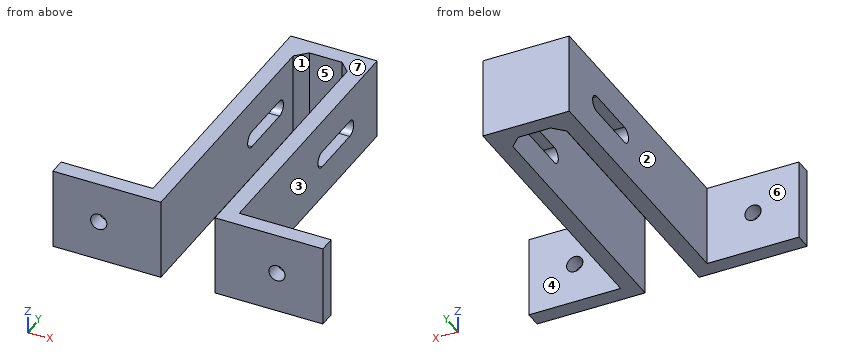
from build123d import *

# Parameters (mm, degrees)
EXTRUDE_1_DEPTH     = 15
SKETCH_2_R          = 1.5
CUT_EXTRUDE_1_DEPTH = 65.210591027
CUT_EXTRUDE_2_DEPTH = 65.210591027
SKETCH_5_R          = 1.5
CUT_EXTRUDE_3_DEPTH = 61.207972894
EXTRUDE_2_DEPTH     = 15


with BuildPart() as part:
    # 草图1 → 凸台-拉伸1 (new body)
    with BuildSketch(Plane.XY):
        Polygon((0, 0), (0, 50), (10, 50), (10, 0), (30, 0), (30, 3), (13, 3), (13, 53), (-3, 53), (-3, 3), (-20, 3), (-20, 0), align=None)
    extrude(amount=EXTRUDE_1_DEPTH)

    # 草图2 → 切除-拉伸1 (cut, through all)
    with BuildSketch(Plane(origin=(13, 0, 0), x_dir=(0, 0, -1), z_dir=(1, 0, 0))):
        with Locations((-7.5, 43)):
            Circle(SKETCH_2_R)
    extrude(amount=-CUT_EXTRUDE_1_DEPTH, mode=Mode.SUBTRACT)

    # 草图4 → 切除-拉伸2 (cut, through all)
    with BuildSketch(Plane(origin=(13, 0, 0), x_dir=(0, 0, -1), z_dir=(1, 0, 0))):
        with BuildLine():
            ThreePointArc((-6, 43), (-7.5, 41.5), (-9, 43))
            Line((-9, 43), (-9, 33))
            ThreePointArc((-9, 33), (-7.5, 34.5), (-6, 33))
            Line((-6, 33), (-6, 43))
        make_face()
        with BuildLine():
            ThreePointArc((-6, 33), (-7.5, 34.5), (-9, 33))
            Line((-9, 33), (-6, 33))
        make_face()
        with BuildLine():
            Line((-6, 33), (-9, 33))
            ThreePointArc((-9, 33), (-7.5, 31.5), (-6, 33))
        make_face()
    extrude(amount=-CUT_EXTRUDE_2_DEPTH, mode=Mode.SUBTRACT)

    # 草图5 → 切除-拉伸3 (cut, through all)
    with BuildSketch(Plane(origin=(0, 3, 0), x_dir=(1, 0, 0), z_dir=(0, 1, 0))):
        with Locations(Location((-11.5, -7.5, 0), (0, 0, 270))):
            Circle(SKETCH_5_R)
        with Locations(Location((21.5, -7.5, 0), (0, 0, 270))):
            Circle(SKETCH_5_R)
    extrude(amount=-CUT_EXTRUDE_3_DEPTH, mode=Mode.SUBTRACT)

    # 草图6 → 凸台-拉伸2 (add)
    with BuildSketch(Plane.XY.offset(15)):
        Polygon((0, 50), (2, 50), (0, 48), align=None)
        Polygon((10, 50), (8, 50), (10, 48), align=None)
    extrude(amount=-EXTRUDE_2_DEPTH)


solid = part.part
Read the model definition and answer for the solid it produces. Units are mm, in the model's axes. Face numbers are marked on the shaded views. A direction names the side the tool comes from. Round coordinates to 2 decimals unless told otherwise and drop trailing zeros. Order: outer loops, then holes, each group sorted by start corner. A loop starts at its lowest first (then second) coordinate and runs counter-clockwise, first axis right, second up.
1) The mould has two halves that part along X. Classify the marked faces 1, 2 and 3: released by +X, released by -X, zero draft, split by the parting line, or undercut.
2) The part is cut by section D-D on z = 11.5. Write down the section's boundary in (x, y), plus the area to 3 significant figures.
3) The part is cut by section C-C on x = -11.5. Write down the section's boundary in (y, z).
4) For the marked faces 4, 5, 6 and 7, determine the directions among +Z, -Z, +X, -X, +Y, -Y from which every point of the face is accessible in a straight line to the end or side of a thin tool.
5) Flat-ended cylindrical pins translate along their axes: pin 1 (4.5 mm diameter, centred on x = -11.5, z = 6.5, fed in from +Y); pin 2 (4.5 mm diameter, centred on y = 39.5, z = 8.5, fed in from -X); pin 3 (3 mm diameter, centred on x = 5.5, z = 7, fed in from -Y). Find the tip coordinate at first contact, or state that the pin passes through.
6) The part is cut by section A-A on z = 7.5. Give the number of separate pieces and of enclosed holes in the cut face, plus the area to 3 significant figures.
7) Straight lines are drawn through the part: L1, parallel to X at y = 0.8, z = 7.5; L2, parallel to X at y = 11.5, z = 6; L3, parallel to Y at x = 22, z = 4.75. For each, find the intervals that lie inside material, in ascending order.
8) The part is cut by section B-B on y = 29.5. Write down the section's boundary in (x, z).
Resolved:
1. face 1: undercut
1. face 2: released by -X
1. face 3: released by +X
2. outline: (-20, 0) - (0, 0) - (0, 48) - (2, 50) - (8, 50) - (10, 48) - (10, 0) - (30, 0) - (30, 3) - (13, 3) - (13, 53) - (-3, 53) - (-3, 3) - (-20, 3) - close
2. area: 454 mm2
3. outline: (0, 0) - (3, 0) - (3, 6) - (0, 6) - close; (0, 9) - (3, 9) - (3, 15) - (0, 15) - close
4. face 4: +Z, -Z, +X, +Y
4. face 5: +Z, -Z, -Y
4. face 6: +Z, -Z, -X, +Y
4. face 7: +Z, +X, -X, +Y, -Y
5. pin 1: stops at y = 3
5. pin 2: stops at x = -3
5. pin 3: stops at y = 50
6. separate pieces: 5
6. enclosed holes: 0
6. area: 358 mm2
7. L1: x = -20 to -13, -10 to 0, 10 to 20, 23 to 30
7. L2: x = -3 to 0, 10 to 13
7. L3: y = 0 to 3
8. outline: (-3, 0) - (0, 0) - (0, 15) - (-3, 15) - close; (10, 0) - (13, 0) - (13, 15) - (10, 15) - close
